Design review of the part shown in the three views and the two pictorial views. Dimensions are in mm from the part's minimum x, y and z. A direction names the side the tool comes from. Round coordinates to 2 decimals unless told otherwise and drop trailing zeros. Loops run counter-clockwise (first coordinate to the right, second up) from the corner with the lowest first, then second, coordinate; pieces in that order, holes last.
1. To check wall thickness, follow line 1 along Z through (x, y) = (22, 9.5); line 2 along Y through (x, z) = (15, 9.75); line 3 along Z through (x, y) = (10, 25.5). State the ranges of each line that lie inside material, in increasing order.
2. Consider section B-B on y = 3. State the section outline as (x, z) points.
3. Consider section D-D on x = 8. State the section outline as (y, z) points, then the cut area to 3 significant figures.
4. Tool access review of the marked faces 4, 5 and 6: name each direction out of +Z, -Z, +X, -X, +Y, -Y from which nothing blocks a thin tool from reaching the whole face with its end or side.
5. Clearance check with flat-ended pins moving along their axes: pin 1 Ø5.5 at (x, z) = (22, 6) entering from +Y; pin 2 Ø7 at (x, z) = (8, 6) entering from +Y; pin 3 Ø6.5 at (x, y) = (13, 35.5) entering from -Z. State where each tip first meets the part, or that it passes through.
6. Draft analysis for pull direction X (two halves, no side actions). For the marked faces 1, 2 and 3, state which applies: released by +X, released by -X, zero draft, split by the parting line, or undercut.
7. Consider section C-C on z = 10.5. State the section outline as (x, y) points, then the cut area to 3 significant figures.
8. Consider section A-A on x = 15. State the section outline as (y, z) points.
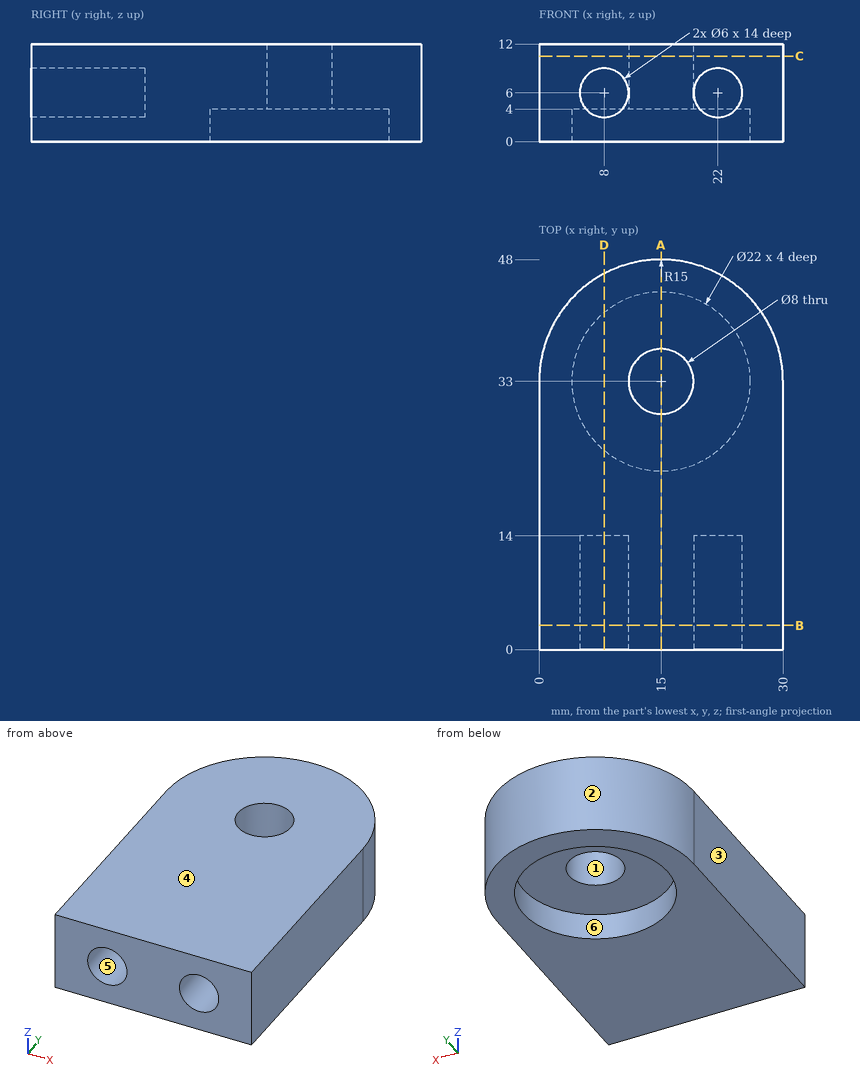
Resolved:
1. line 1: z = 0 to 3, 9 to 12
1. line 2: y = 0 to 29, 37 to 48
1. line 3: z = 4 to 12
2. outline: (0, 0) - (30, 0) - (30, 12) - (0, 12) - close; hole circle Ø6 at (8, 6); hole circle Ø6 at (22, 6)
3. outline: (0, 0) - (24.51, 0) - (24.51, 4) - (41.49, 4) - (41.49, 0) - (46.27, 0) - (46.27, 12) - (0, 12) - (0, 9) - (14, 9) - (14, 3) - (0, 3) - close
3. area: 403 mm2
4. face 4: +Z, +X, -X, +Y, -Y
4. face 5: -Y
4. face 6: -Z
5. pin 1: stops at y = 47.39
5. pin 2: stops at y = 47.59
5. pin 3: stops at z = 4
6. face 1: undercut
6. face 2: split by the parting line
6. face 3: released by -X
7. outline: (0, 0) - (30, 0) - (30, 33) arc R15 ccw to (0, 33) - close; hole circle Ø8 at (15, 33)
7. area: 1,290 mm2
8. outline: (0, 0) - (22, 0) - (22, 4) - (29, 4) - (29, 12) - (0, 12) - close; (37, 4) - (44, 4) - (44, 0) - (48, 0) - (48, 12) - (37, 12) - close
